The model under review builds one solid part; all positions refer to its coordinate system, in mm. Face numbers are marked on the shaded views. A direction names the side the tool comes from. Coordinates: 2 decimals unless noted, no trailing zeros. Loops run counter-clockwise (first coordinate to the right, second up) from the corner with the lowest first, then second, coordinate; pieces in that order, holes last. Notation, with made-up numbers: M 7,58 L 50,58 A24 ccw 50,84 Z; hole C 46.5,9.25 d9. An arc over 180 degrees is marked long. Write item = value, one per line. Start each with the question number.
Q1. We need section C-C on x = -106. Give the boundary of the cut face in (y, z).
Q2. We need section A-A on y = -77. Give the boundary of the cut face in (x, z), and give its area (3 significant figures).
Q3. For the marked faces 1 and 2, list the 3-axis set-ups (+Z, -Z, +X, -X, +Y, -Y) from which the entire face can be reached by the end or side of a thin tool; tool diameter is ignored.
Q4. Wall thickness on probe 1 along X at (y, z) = (-74.5, 6.85); probe 2 along X at (y, z) = (-79, 5.7); probe 3 along Y at (x, z) = (-101.5, 5.15): over which ranges is each line inside the solid? List them lowest first.
Q5. We need section B-B on z = 6.6. Give the boundary of the cut face in (x, y) (3 decimals), and give its area (3 significant figures).
Q6. Mouldability with a two-part tool opening along Y and no side actions: class the marked faces 3, 4, 5 and 6 as released by +Y, released by -Y, zero draft, split by the parting line, or undercut.
Q7. Clearance check with a flat-ended pin moving along its axis: pin 1 Ø1 at (x, z) = (-123, 6) entering from -Y. State where the tip first meets the part, or that it passes through.
Q8. We need section D-D on x = -129. Give the boundary of the cut face in (y, z).
from build123d import *

# Parameters (mm, degrees)
BOSS_EXTRUDE3_START = 4.7625
BOSS_EXTRUDE3_DEPTH = 2.54


with BuildPart() as part:
    # Sketch2 → Boss-Extrude3 (new body)
    with BuildSketch(Plane.XY.offset(BOSS_EXTRUDE3_START)):
        with BuildLine():
            Line((-132.173225325, -84.582396488), (-112.918972687, -67.080031215))
            ThreePointArc((-112.918972687, -67.080031215), (-94.978825746, -67.935091298), (-95.833885829, -85.875238239))
            Line((-95.833885829, -85.875238239), (-115.088138468, -103.377603512))
            ThreePointArc((-115.088138468, -103.377603512), (-114.233078385, -85.437456571), (-132.173225325, -84.582396488))
        make_face()
        with BuildLine():
            Line((-107.551429258, -79.652634727), (-101.201429258, -79.652634727))
            ThreePointArc((-101.201429258, -79.652634727), (-98.026429258, -76.477634727), (-101.201429258, -73.302634727))
            Line((-101.201429258, -73.302634727), (-107.551429258, -73.302634727))
            ThreePointArc((-107.551429258, -73.302634727), (-110.726429258, -76.477634727), (-107.551429258, -79.652634727))
        make_face(mode=Mode.SUBTRACT)
    extrude(amount=BOSS_EXTRUDE3_DEPTH)


solid = part.part
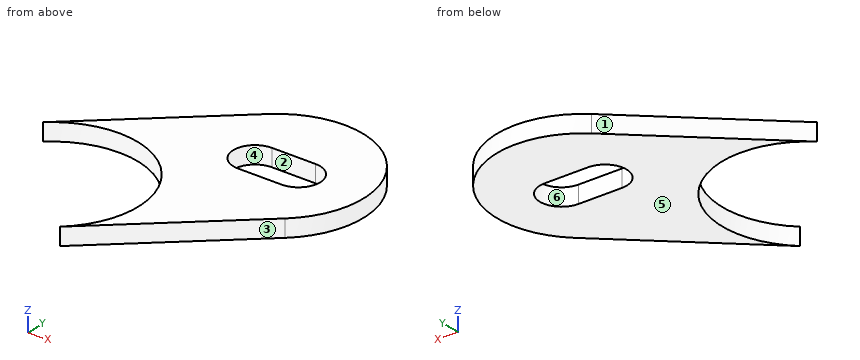
Returned:
q1.outline = M -95.12,4.76 L -79.65,4.76 L -79.65,7.3 L -95.12,7.3 Z; M -73.3,4.76 L -63.88,4.76 L -63.88,7.3 L -73.3,7.3 Z
q2.outline = M -123.83,4.76 L -110.68,4.76 L -110.68,7.3 L -123.83,7.3 Z; M -98.07,4.76 L -91.69,4.76 L -91.69,7.3 L -98.07,7.3 Z
q2.area = 49.6 mm^2
q3.face_1 = +Z, -Z, -X, +Y
q3.face_2 = +Z, -Z
q4.probe_1 = -121.08 to -110.04, -98.72 to -91.83
q4.probe_2 = -126.03 to -109.48, -99.27 to -91.93
q4.probe_3 = -91.03 to -79.65, -73.3 to -64.11
q5.outline = M -132.173,-84.582 A12.7 cw -115.088,-103.378 L -95.834,-85.875 A12.7 ccw -112.919,-67.08 Z; hole M -107.551,-79.653 L -101.201,-79.653 A3.175 ccw -101.201,-73.303 L -107.551,-73.303 A3.175 ccw Z
q5.area = 589 mm^2
q6.face_3 = released by -Y
q6.face_4 = undercut
q6.face_5 = zero draft
q6.face_6 = undercut
q7.pin_1 = -81.33
q8.outline = M -82.47,4.76 L -81.7,4.76 L -81.7,7.3 L -82.47,7.3 Z
